The listing builds one solid part. Answer for the finished solid, in the listing's coordinates (mm). A direction names the side the tool comes from. Give positions to 0.01 mm unless a question says otherwise; leave off trailing zeros. Loops run counter-clockwise (first coordinate to the right, second up) from the corner with the lowest first, then second, coordinate; pieces in that order, holes last. Notation, with made-up numbers: (59, -6.5) - (88, -6.5) arc R19 ccw to (88, 2.5) - close; hole circle Ø6 at (68.5, -14). An arc over 180 degrees is marked (long way). One line per item, written item: value. Start each with the question number.
from build123d import *

# Parameters (mm, degrees)
F0_W     = 101.6
F0_H     = 76.2
F1_DEPTH = 25.4
F2_R     = 6.35
F3_DEPTH = 25.401
F4_W     = 12.7
F4_H     = 12.7
F6_W     = 7.62
F6_H     = 7.1126786113
F8_W     = 12.7
F8_H     = 12.7
F10_R    = 2.54
F11_SIZE = 2.54
F12_R    = 2.54


with BuildPart() as f1:
    # F0 (on Top) → F1 (new body)
    with BuildSketch(Plane.XY):
        Rectangle(F0_W, F0_H)
    extrude(amount=F1_DEPTH)

    # F2 (on face) → F3 (cut, through all)
    with BuildSketch(Plane(origin=(0, 0, 0), x_dir=(1, 0, 0), z_dir=(0, 0, -1))):
        with Locations((31.75, 19.05)):
            Circle(F2_R)
        with Locations((31.75, -19.05)):
            Circle(F2_R)
        with Locations((-31.75, -19.05)):
            Circle(F2_R)
        with Locations((-31.75, 19.05)):
            Circle(F2_R)
    extrude(amount=-F3_DEPTH, mode=Mode.SUBTRACT)

    # F4 (on Front) → F5 (revolve)
    with BuildSketch(Plane.XZ):
        with Locations((6.35, 31.75)):
            Rectangle(F4_W, F4_H)
    revolve(axis=Axis((0, 0, 31.75), (0, 0, 1)))

    # F6 (on Front) → F7 (revolve)
    with BuildSketch(Plane.XZ):
        with Locations((3.81, 41.6563393056)):
            Rectangle(F6_W, F6_H)
    revolve(axis=Axis((0, 0, 41.6563393056), (0, 0, 1)))

    # F8 (on Front) → F9 (revolve)
    with BuildSketch(Plane.XZ):
        with Locations((-6.35, 51.5626786113)):
            Rectangle(F8_W, F8_H)
    revolve(axis=Axis((0, 0, 51.5626786113), (0, 0, -1)))

    # F10
    f10_edges = [f1.edges().sort_by_distance(p)[0] for p in [
        (12.7, 0, 57.912679),
    ]]
    fillet(f10_edges, radius=F10_R)

    # F11
    f11_edges = [f1.edges().sort_by_distance(p)[0] for p in [
        (0, -38.1, 25.4),
        (-50.8, 0, 25.4),
        (0, 38.1, 25.4),
        (50.8, 0, 25.4),
    ]]
    chamfer(f11_edges, length=F11_SIZE)

    # F12
    f12_edges = [f1.edges().sort_by_distance(p)[0] for p in [
        (-12.7, 0, 25.4),
        (-12.7, 0, 38.1),
        (12.7, 0, 45.212679),
    ]]
    fillet(f12_edges, radius=F12_R)


solid = f1.part
1. A cutting plane is placed at A-A (y = 19.05). Determine the outline of the cut face in (x, z).
2. A cutting plane is placed at C-C (z = 7.5). Determine the outline of the cut face in (x, y), plus the area to 3 significant figures.
3. Determine the mould class of faces 1 (the cylindrical face through (-28.336, -24.404, 12.522)), 2 (the cylindrical face through (37.807, -20.957, 12.522)), 3 (the flat face through (-1, 8, 38.1)), 4 (the flat face through (-1, 38.1, 11)) for opening direction Y: released by +Y, released by -Y, zero draft, split by the parting line, or undercut.
4. A cutting plane is placed at D-D (x = 16.5). Determine the outline of the cut face in (y, z), plus the area to 3 significant figures.
5. Flat-ended cylindrical pins translate along their axes: pin 1 (8 mm diameter, centred on y = 12.5, z = 47, fed in from -X); pin 2 (5 mm diameter, centred on y = 4.5, z = 44.5, fed in from +X); pin 3 (10 mm diameter, centred on x = 31.75, y = 19.05, fed in from -Z); pin 4 (12 mm diameter, centred on x = -2.5, y = -26, fed in from +Z). Find the tip coordinate at first contact, or state that the pin passes through.
6. For faces 5 (the cylindrical face through (-1.65, -7.44, 41.71)), 6 (the cylindrical face through (2.75, -12.4, 51.62)), 7 (the flat face through (49.55, -0.53, 24.11)), determine the directions among +Z, -Z, +X, -X, +Y, -Y from which every point of the face is accessible in a straight line to the end or side of a thin tool.
7. A cutting plane is placed at B-B (x = 31.75). Determine the outline of the cut face in (y, z).
8. Find the intervals of material crossed by L1, parallel to Y at x = -31.75, z = 17.25; L2, parallel to X at y = 19.05, z = 19.25; L3, parallel to Y at x = 29, z = 9, in increasing order. Write a range as [from, to].
Results below:
1. outline: (-50.8, 0) - (-38.1, 0) - (-38.1, 25.4) - (-48.26, 25.4) - (-50.8, 22.86) - close; (-25.4, 0) - (25.4, 0) - (25.4, 25.4) - (-25.4, 25.4) - close; (38.1, 0) - (50.8, 0) - (50.8, 22.86) - (48.26, 25.4) - (38.1, 25.4) - close
2. outline: (-50.8, -38.1) - (50.8, -38.1) - (50.8, 38.1) - (-50.8, 38.1) - close; hole circle Ø12.7 at (-31.75, -19.05); hole circle Ø12.7 at (-31.75, 19.05); hole circle Ø12.7 at (31.75, -19.05); hole circle Ø12.7 at (31.75, 19.05)
2. area: 7,240 mm^2
3. face 1: undercut
3. face 2: undercut
3. face 3: zero draft
3. face 4: released by +Y
4. outline: (-38.1, 0) - (38.1, 0) - (38.1, 22.86) - (35.56, 25.4) - (-35.56, 25.4) - (-38.1, 22.86) - close
4. area: 1,930 mm^2
5. pin 1: stops at x = -9.39
5. pin 2: stops at x = 12.02
5. pin 3: passes through
5. pin 4: stops at z = 25.4
6. face 5: none
6. face 6: +Z
6. face 7: +Z, +X, +Y, -Y
7. outline: (-38.1, 0) - (-25.4, 0) - (-25.4, 25.4) - (-35.56, 25.4) - (-38.1, 22.86) - close; (-12.7, 0) - (12.7, 0) - (12.7, 25.4) - (-12.7, 25.4) - close; (25.4, 0) - (38.1, 0) - (38.1, 22.86) - (35.56, 25.4) - (25.4, 25.4) - close
8. L1: y = [-38.1, -25.4], [-12.7, 12.7], [25.4, 38.1]
8. L2: x = [-50.8, -38.1], [-25.4, 25.4], [38.1, 50.8]
8. L3: y = [-38.1, -24.77], [-13.33, 13.33], [24.77, 38.1]
